Part print with two shaded views. Sizes in mm from the minimum x, y, z corner. Give positions to 0.01 mm unless a question says otherwise; leave off trailing zeros. Order: outer loops, then holes, each group sorted by start corner. A loop starts at its lowest first (then second) coordinate and runs counter-clockwise, first axis right, second up. Notation, with made-up numbers: M -33,-38 L -19,-38 A24 cw -19,-8 Z; hole C 74,53.25 d7. An arc over 180 degrees is marked long. Return JSON: item names as keys, results as strings. Group by question number.
1. Slice it at B-B on z = 60. List the corners of the cut face in (x, y).
2. Pin check, flat tips, straight feed: pin 1 (1 mm diameter, centred on x = 41, y = 1, fed in from -Z); pin 2 (5 mm diameter, centred on x = 80, y = 2, fed in from +Z); pin 3 (3 mm diameter, centred on x = 82.5, y = 2.5, fed in from -Z) (3 decimals); pin 4 (4.5 mm diameter, centred on x = 19, z = 60, fed in from +Y). Stop position of each tip, or through.
3. Wall check: probe 1 along Z at (x, y) = (101, 5); probe 2 along X at (y, z) = (3.75, 85.5); probe 3 along X at (y, z) = (2.75, 113.5). Give the ranges that are in metal, low to high. Write a range as [from, to].
4. Slice it at C-C on x = 39. List the corners of the cut face in (y, z).
5. Two-plate mould, pull along Z, no slides. Class the marked faces 1, 2 and 3: released by +Z, released by -Z, zero draft, split by the parting line, or undercut.
6. Slice it at D-D on z = 89.5. List the corners of the cut face in (x, y).
7. Slice it at A-A on y = 5.5. Give the number of separate pieces and of enclosed holes in the cut face, then the cut area to 3 significant figures.
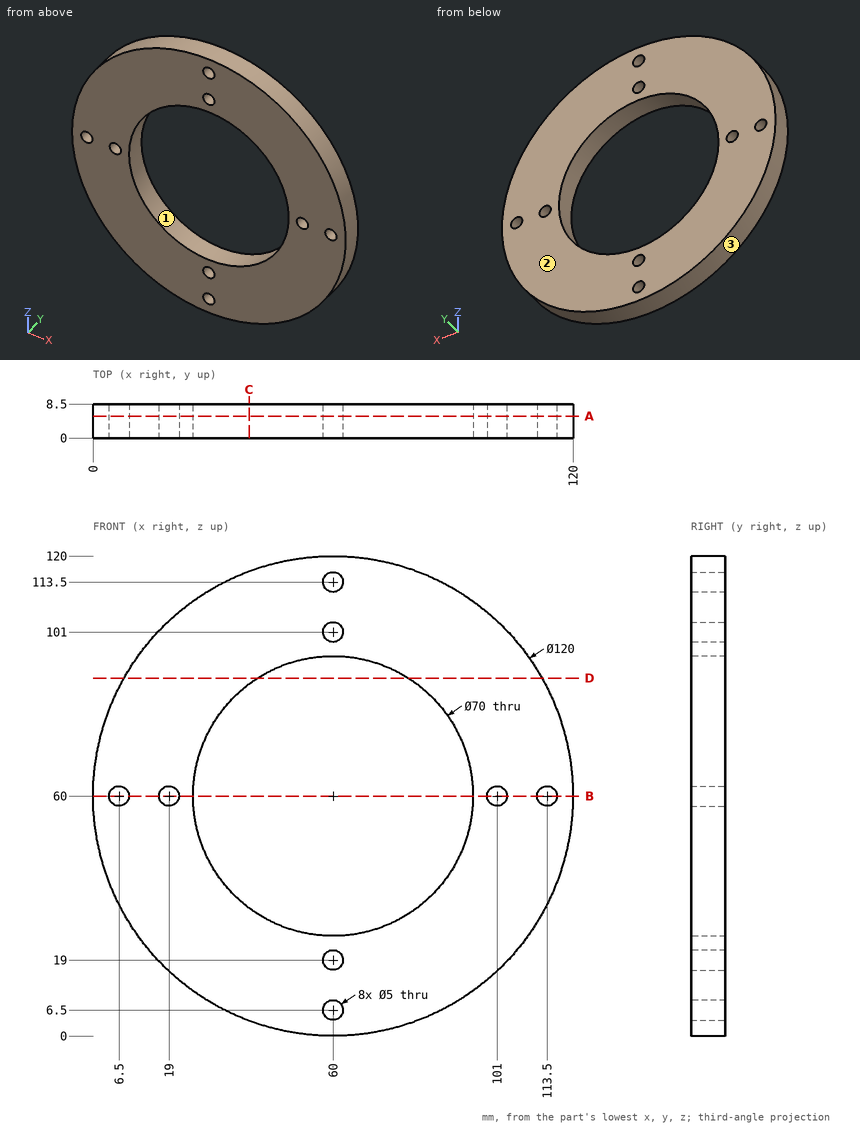
Result:
{
 "1": {"outline": "M 0,0 L 4,0 L 4,8.5 L 0,8.5 Z; M 9,0 L 16.5,0 L 16.5,8.5 L 9,8.5 Z; M 21.5,0 L 25,0 L 25,8.5 L 21.5,8.5 Z; M 95,0 L 98.5,0 L 98.5,8.5 L 95,8.5 Z; M 103.5,0 L 111,0 L 111,8.5 L 103.5,8.5 Z; M 116,0 L 120,0 L 120,8.5 L 116,8.5 Z"},
 "2": {"pin 1": "stops at z = 2.92", "pin 2": "stops at z = 117.39", "pin 3": "stops at z = 3.795", "pin 4": "passes through"},
 "3": {"probe 1": "z = [16.19, 57.5], [62.5, 103.81]", "probe 2": "x = [5.69, 36.03], [83.97, 114.31]", "probe 3": "x = [32.84, 57.5], [62.5, 87.16]"},
 "4": {"outline": "M 0,3.8 L 8.5,3.8 L 8.5,32 L 0,32 Z; M 0,88 L 8.5,88 L 8.5,116.2 L 0,116.2 Z"},
 "5": {"face 1": "undercut", "face 2": "zero draft", "face 3": "split by the parting line"},
 "6": {"outline": "M 7.75,0 L 41.17,0 L 41.17,8.5 L 7.75,8.5 Z; M 78.83,0 L 112.25,0 L 112.25,8.5 L 78.83,8.5 Z"},
 "7": {"separate pieces": "1", "enclosed holes": "9", "area": "7,300 mm2"}
}
